Solid Edge part; units mm, degrees
sketch "Sketch1" plane through (0, 0, 0) normal (0, -1, 0) x (1, 0, 0)
  line L0 (9, 5.1962) -> (0, 10.3923)
  line L1 (0, 10.3923) -> (-9, 5.1962)
  line L2 (-9, 5.1962) -> (-9, -5.1962)
  line L3 (-9, -5.1962) -> (0, -10.3923)
  line L4 (0, -10.3923) -> (9, -5.1962)
  line L5 (9, -5.1962) -> (9, 5.1962)
extrude "Protrusion1" add sketch "Sketch1" along normal mid plane 12.2
sketch "Sketch2" plane through (0, 0, 0) normal (1, 0, 0) x (0, 1, 0)
  line L0 (-6.1, 8.25) -> (-5.526, 10.3923)
revolve "RevolvedCutout1" cut sketch "Sketch2" angle 360 about axis through (0, 0, 0) along (0, -1, 0) material side at (0, -5.8613, 9.3341)
mirror "Mirror1" about plane through (0, 0, 0) normal (0, -1, 0) of "RevolvedCutout1"
hole "孔_7" at (0, -6.1, 0) direction (0, 1, 0) diameter 10.106 end up to next start chamfer 1.2 start chamfer angle 60 end chamfer 1.2 end chamfer angle 60
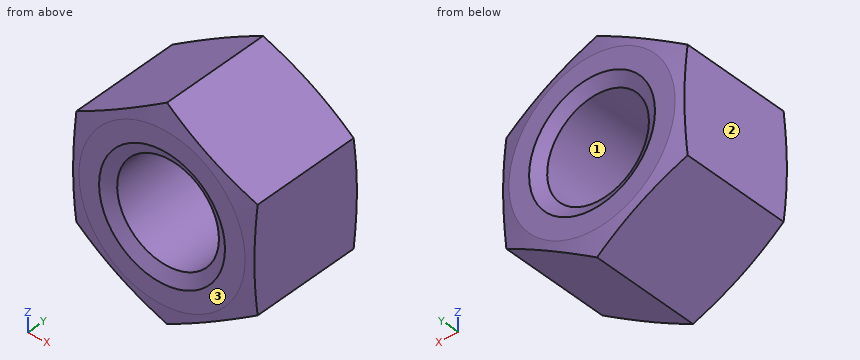
The listing builds one solid part. Answer for the finished solid, in the listing's coordinates (mm). Face numbers are marked on the shaded views. Give positions to 0.01 mm unless a question says otherwise; leave off trailing zeros. Loops run counter-clockwise (first coordinate to the right, second up) from the corner with the lowest first, then second, coordinate; pieces in that order, holes last. Notation, with made-up numbers: M 8,75.5 L 49,75.5 A11 cw 49,89.5 Z; hole C 59,67 d5. An arc over 180 degrees is marked long. One line per item, written item: value.
1. For a pull along X with two mould halves and no side action, classify the marked faces 1, 2 and 3 as pulls with the +X half, pulls with the -X half, needs draft (parallel to the pull), parting line crosses it, or undercut.
Found:
face 1: undercut
face 2: pulls with the -X half
face 3: needs draft
2. Section B-B on y = -1.25 is taken. Determine the outline of the cut face in (x, z), plus the area to 3 significant figures.
Found:
outline: M -9,-5.2 L 0,-10.39 L 9,-5.2 L 9,5.2 L 0,10.39 L -9,5.2 Z; hole C 0,0 d10.11
area: 200 mm^2
3. Find the intervals of material crossed by probe 1 along X at (y, z) = (-1.25, 0); probe 2 along Z at (x, y) = (1.75, -1.5); probe 3 along Z at (x, y) = (4.5, 3), in increasing order.
Found:
probe 1: -9 to -5.05, 5.05 to 9
probe 2: -9.38 to -4.74, 4.74 to 9.38
probe 3: -7.79 to -2.3, 2.3 to 7.79
4. Section A-A on z = 0 is taken. Determine the outline of the cut face in (x, y).
Found:
outline: M -9,-5.9 L -8.25,-6.1 L -6.25,-6.1 L -5.05,-5.41 L -5.05,5.41 L -6.25,6.1 L -8.25,6.1 L -9,5.9 Z; M 5.05,-5.41 L 6.25,-6.1 L 8.25,-6.1 L 9,-5.9 L 9,5.9 L 8.25,6.1 L 6.25,6.1 L 5.05,5.41 Z
5. Each of these flat-tipped pins is pushed along its axis until it touches: P1, Ø6, axis at x = -3.5, y = 1.5, coming from the +Z side; P2, Ø1.5, axis at x = -4.5, y = -1.5, coming from the +Z side; P3, Ø5, axis at x = -1, z = -3.5, coming from the -Y side. Where does it stop, or does it pass through?
Found:
P1: z = 10.1
P2: z = 8.23
P3: y = -6.03
